```python
from build123d import *

# Parameters (mm, degrees)
CORTAR_EXTRUIR1_DEPTH = 128.279220614


with BuildPart() as part:
    # Croquis1 → Revolución1 (revolve)
    with BuildSketch(Plane(origin=(0, 0, 0), x_dir=(1, 0, 0), z_dir=(0, 1, 0)), mode=Mode.PRIVATE) as revoluci_n1_sk:
        Polygon((0, 55.393258427), (-30, 55.393258427), (-30, 35.393258427), (-25.4, 35.393258427), (-25.4, -44.606741573), (-30, -44.606741573), (-30, -64.606741573), (0, -64.606741573), align=None)
    revolve(revoluci_n1_sk.sketch.rotate(Axis((0, 0, 64.606741573), (0, 0, -1)), 180), axis=Axis((0, 0, 64.606741573), (0, 0, -1)))

    # Croquis2 → Cortar-Extruir1 (cut, through all)
    with BuildSketch(Plane(origin=(0, 0, -55.393258427), x_dir=(-1, 0, 0), z_dir=(0, 0, -1))):
        Polygon((7.332348419, 0), (3.666174209, 6.35), (-3.666174209, 6.35), (-7.332348419, 0), (-3.666174209, -6.35), (3.666174209, -6.35), align=None)
    extrude(amount=-CORTAR_EXTRUIR1_DEPTH, mode=Mode.SUBTRACT)


solid = part.part
```
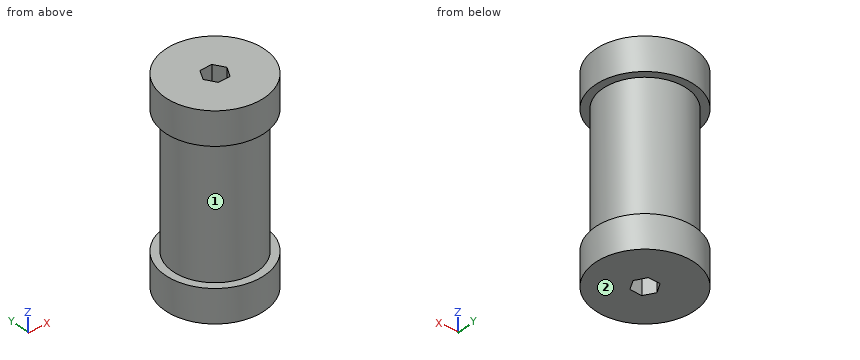
Can you work these out from the model? Positions are in its coordinate system, mm. Face numbers are marked on the shaded views. A direction names the side the tool comes from. Coordinates: 2 decimals unless noted, no trailing zeros. Order: outer loops, then holes, each group sorted by start corner. A loop starts at its lowest first (then second) coordinate and runs counter-clockwise, first axis right, second up. Notation, with made-up numbers: (54, 34) -> (91, 34) arc R22 cw to (91, 66) -> close; hole circle Ø6 at (5.5, -8). An arc over 180 degrees is marked (long way). Write each question's results on one line, items separated by ' | '.
Item 1: I want a section at C-C, the plane y = -13. Write out the boundary of the cut face in (x, z).
Results are:
outline: (-27.04, -55.39) -> (27.04, -55.39) -> (27.04, -35.39) -> (21.82, -35.39) -> (21.82, 44.61) -> (27.04, 44.61) -> (27.04, 64.61) -> (-27.04, 64.61) -> (-27.04, 44.61) -> (-21.82, 44.61) -> (-21.82, -35.39) -> (-27.04, -35.39) -> close
Item 2: I'm going to push flat-ended pins straight in: pin 1 Ø1 at (x, z) = (-9, 42) entering from +Y; pin 2 Ø2 at (x, z) = (1, -0.5) entering from -Y; pin 3 Ø5 at (y, z) = (12.5, -7) entering from -X. Where does each tip first touch, or does it pass through?
Results are:
pin 1: y = 23.94 | pin 2: y = -25.4 | pin 3: x = -23.35
Item 3: Which directions (+Z, -Z, +X, -X, +Y, -Y) give clear straight access to the entire face, cutting with the end or side of a thin tool? Please do the marked faces 1 and 2.
Results are:
face 1: none | face 2: -Z, +X, -X, +Y, -Y
Item 4: If I drill on line 1 along Z through (x, y) = (-26.5, 1); line 2 along Y through (x, z) = (2, 54); line 3 along X through (y, z) = (-3, -5), over which ranges is the centre line in solid material (lowest first)?
Results are:
line 1: -55.39 to -35.39, 44.61 to 64.61 | line 2: -29.93 to -6.35, 6.35 to 29.93 | line 3: -25.22 to -5.6, 5.6 to 25.22
Item 5: I want a section at B-B, the plane x = 6. Write out the boundary of the cut face in (y, z).
Results are:
outline: (-29.39, -55.39) -> (-2.31, -55.39) -> (-2.31, 64.61) -> (-29.39, 64.61) -> (-29.39, 44.61) -> (-24.68, 44.61) -> (-24.68, -35.39) -> (-29.39, -35.39) -> close; (2.31, -55.39) -> (29.39, -55.39) -> (29.39, -35.39) -> (24.68, -35.39) -> (24.68, 44.61) -> (29.39, 44.61) -> (29.39, 64.61) -> (2.31, 64.61) -> close
Item 6: I want a section at D-D, the plane x = -22. Write out the boundary of the cut face in (y, z).
Results are:
outline: (-20.4, -55.39) -> (20.4, -55.39) -> (20.4, -35.39) -> (12.69, -35.39) -> (12.69, 44.61) -> (20.4, 44.61) -> (20.4, 64.61) -> (-20.4, 64.61) -> (-20.4, 44.61) -> (-12.69, 44.61) -> (-12.69, -35.39) -> (-20.4, -35.39) -> close
Item 7: I want a section at A-A, the plane z = -43. Write out the boundary of the cut face in (x, y).
Results are:
outline: circle Ø60 at (0, 0); hole (-7.33, 0) -> (-3.67, -6.35) -> (3.67, -6.35) -> (7.33, 0) -> (3.67, 6.35) -> (-3.67, 6.35) -> close
